```python
from build123d import *

# Parameters (mm, degrees)
SKETCH_1_W          = 27.799055089
SKETCH_1_H          = 170
SKETCH_1_R          = 1.5
EXTRUDE_1_DEPTH     = 5
EXTRUDE_2_DEPTH     = 170
FILLET_1_R          = 20
FILLET_2_R          = 20
SKETCH_3_R          = 1.5
CUT_EXTRUDE_1_DEPTH = 22
SKETCH_5_W          = 53.411136204
SKETCH_5_H          = 30.531921538
CUT_EXTRUDE_2_DEPTH = 138
SKETCH_6_W          = 16.9901426
SKETCH_6_H          = 53.411136204
EXTRUDE_3_DEPTH     = 7.098148729
FILLET_3_R          = 2
SKETCH_7_R          = 1.5
CUT_EXTRUDE_3_DEPTH = 20


with BuildPart() as part:
    # 草图1 → 凸台-拉伸1 (new body)
    with BuildSketch(Plane(origin=(0, 0, 0), x_dir=(1, 0, 0), z_dir=(0, 1, 0))):
        with Locations((91.881203353, 5)):
            Rectangle(SKETCH_1_W, SKETCH_1_H)
        with Locations(Location((82.140918425, 87.25, 0), (0, 0, 270))):
            Circle(SKETCH_1_R, mode=Mode.SUBTRACT)
        with Locations(Location((92.640918425, 87.25, 0), (0, 0, 270))):
            Circle(SKETCH_1_R, mode=Mode.SUBTRACT)
        with Locations(Location((82.140918425, -77.25, 0), (0, 0, 270))):
            Circle(SKETCH_1_R, mode=Mode.SUBTRACT)
        with Locations(Location((92.640918425, -77.25, 0), (0, 0, 270))):
            Circle(SKETCH_1_R, mode=Mode.SUBTRACT)
    extrude(amount=EXTRUDE_1_DEPTH)

    # 草图2 → 凸台-拉伸2 (add)
    with BuildSketch(Plane.XY.offset(80)):
        Polygon((70.154089187, 3.11568229), (59.601778844, 32.107916678), (60.432470808, 37.577633674), (62.77468262, 53), (74.6026601, 53), (68.115201024, 32.107916678), (77.981675808, 5), (77.981675808, 0), (71.288104799, 0), align=None)
    extrude(amount=-EXTRUDE_2_DEPTH)

    # 圆角1
    fillet_1_edges = [part.edges().sort_by_distance(p)[0] for p in [
        (59.601778844, 32.107916678, -5),
    ]]
    fillet(fillet_1_edges, radius=FILLET_1_R)

    # 圆角2
    # the kernel refuses this fillet: 20 mm, written as the material it takes off along each edge
    with BuildSketch(Plane(origin=(71.288104799, 0, 115.01037691), x_dir=(-0.34202014332567304, 0.9396926207859069, 0), z_dir=(0, 0, -1))) as fillet_2_piece_1:
        with BuildLine():
            CenterArc((FILLET_2_R * 0.70020753821, FILLET_2_R), FILLET_2_R, 200, 70)
            Line((-FILLET_2_R * 0.239485082576, FILLET_2_R * 0.657979856674), (0, 0))
            Line((0, 0), (FILLET_2_R * 0.70020753821, 0))
        make_face()
    extrude(amount=240.020753821, mode=Mode.SUBTRACT)

    # 草图3 → 切除-拉伸1 (cut)
    with BuildSketch(Plane(origin=(0, 53, 0), x_dir=(1, 0, 0), z_dir=(0, 1, 0))):
        with Locations(Location((71.288104799, 70.02483454, 0), (0, 0, 270))):
            Circle(SKETCH_3_R)
        with Locations(Location((65.841750728, 62.078973455, 0), (0, 0, 270))):
            Circle(SKETCH_3_R)
        with Locations(Location((65.841750728, 55.078973455, 0), (0, 0, 270))):
            Circle(SKETCH_3_R)
        with Locations(Location((71.288104799, 47.133112371, 0), (0, 0, 270))):
            Circle(SKETCH_3_R)
        with Locations(Location((71.288104799, -37.133112371, 0), (0, 0, 270))):
            Circle(SKETCH_3_R)
        with Locations(Location((65.841750728, -45.078973455, 0), (0, 0, 270))):
            Circle(SKETCH_3_R)
        with Locations(Location((65.841750728, -52.078973455, 0), (0, 0, 270))):
            Circle(SKETCH_3_R)
        with Locations(Location((71.288104799, -60.02483454, 0), (0, 0, 270))):
            Circle(SKETCH_3_R)
    extrude(amount=-CUT_EXTRUDE_1_DEPTH, mode=Mode.SUBTRACT)

    # 草图5 → 切除-拉伸2 (cut)
    with BuildSketch(Plane(origin=(0, 0, 0), x_dir=(0, 0, -1), z_dir=(1, 0, 0))):
        with Locations((5, 27.364109498)):
            Rectangle(SKETCH_5_W, SKETCH_5_H)
    extrude(amount=CUT_EXTRUDE_2_DEPTH, mode=Mode.SUBTRACT)

    # 草图6 → 凸台-拉伸3 (add)
    with BuildSketch(Plane(origin=(0, 5, 0), x_dir=(1, 0, 0), z_dir=(0, 1, 0))):
        with Locations((83.893232252, 5)):
            Rectangle(SKETCH_6_W, SKETCH_6_H)
    extrude(amount=EXTRUDE_3_DEPTH)

    # 圆角3
    fillet_3_edges = [part.edges().sort_by_distance(p)[0] for p in [
        (71.158795105, 12.098148729, -31.705568102),
        (71.158795105, 12.098148729, 21.705568102),
        (66.291177476, 42.630070267, 21.705568102),
        (66.291177476, 42.630070267, -31.705568102),
    ]]
    fillet(fillet_3_edges, radius=FILLET_3_R)

    # 草图7 → 切除-拉伸3 (cut)
    with BuildSketch(Plane(origin=(0, 12.098148729, 0), x_dir=(1, 0, 0), z_dir=(0, 1, 0))):
        with Locations(Location((71.530354556, -14, 0), (0, 0, 270))):
            Circle(SKETCH_7_R)
        with Locations(Location((71.530354556, 24, 0), (0, 0, 270))):
            Circle(SKETCH_7_R)
        with Locations(Location((86.530354556, 24, 0), (0, 0, 270))):
            Circle(SKETCH_7_R)
        with Locations(Location((86.530354556, -14, 0), (0, 0, 270))):
            Circle(SKETCH_7_R)
    extrude(amount=-CUT_EXTRUDE_3_DEPTH, mode=Mode.SUBTRACT)


solid = part.part
```
Can you work these out from the model? Positions are in its coordinate system, mm. A direction names the side the tool comes from. Give positions to 0.01 mm unless a question says otherwise; leave off trailing zeros. Write each loop counter-clockwise with the first axis right and the second up, starting at its lowest first coordinate (ties: lowest second). Pieces come first, ordered by that corner, then holes. Notation, with made-up numbers: (74, 24) -> (133, 24) arc R15 ccw to (133, 37) -> close; hole circle Ø4 at (26, -36.75). An arc over 180 degrees is marked (long way). One line per item, written item: value.
Q1. Imagine slicing it at B-B on z = 77.25. Please give me the cut outline in (x, y).
Results found:
outline: (60.37, 37.15) arc R20 ccw to (61.35, 27.31) -> (66.5, 13.16) arc R20 ccw to (80.64, 0.55) -> (80.64, 5) -> (77.98, 5) -> (68.12, 32.11) -> (74.6, 53) -> (62.77, 53) -> close; (83.64, 0.07) arc R20 ccw to (85.29, 0) -> (91.14, 0) -> (91.14, 5) -> (83.64, 5) -> close; (94.14, 0) -> (105.78, 0) -> (105.78, 5) -> (94.14, 5) -> close
Q2. Imagine slicing it at A-A on y = 46. Please give me the cut outline in (x, z).
Results found:
outline: (61.71, -90) -> (72.43, -90) -> (72.43, -71) arc R1.5 cw (long way) to (72.43, -69.05) -> (72.43, -48.11) arc R1.5 cw (long way) to (72.43, -46.16) -> (72.43, 36.16) arc R1.5 cw (long way) to (72.43, 38.11) -> (72.43, 59.05) arc R1.5 cw (long way) to (72.43, 61) -> (72.43, 80) -> (61.71, 80) -> close; hole circle Ø3 at (65.84, -62.08); hole circle Ø3 at (65.84, -55.08); hole circle Ø3 at (65.84, 45.08); hole circle Ø3 at (65.84, 52.08)
Q3. Which directions (+Z, -Z, +X, -X, +Y, -Y) give clear straight access to the entire face, cutting with the end or side of a thin tool? Please do faces 1 (the face through (60.247, 32.102, 50.445)), 2 (the face through (73.018, 9.082, 13.805)), 3 (the face through (84, 8, 21.706)), 4 (the face through (64.51, 42.15, 45.77)).
Results found:
face 1: +Z, -Z, -X
face 2: -Y
face 3: +Z, +X, +Y
face 4: +Y
Q4. Imagine slicing it at C-C on x = 96. Please give me the cut outline in (y, z).
Results found:
outline: (0, -90) -> (5, -90) -> (5, 80) -> (0, 80) -> close
Q5. Imagine slicing it at D-D on y = 9. Please give me the cut outline in (x, z), and give its area (3 significant figures).
Results found:
outline: (68.59, -90) -> (76.53, -90) -> (76.53, -31.71) -> (92.39, -31.71) -> (92.39, 21.71) -> (76.53, 21.71) -> (76.53, 80) -> (68.59, 80) -> close; hole circle Ø3 at (71.53, -24); hole circle Ø3 at (71.53, 14); hole circle Ø3 at (86.53, -24); hole circle Ø3 at (86.53, 14)
area: 2,170 mm^2
Q6. We'd pull the mould along X, two halves only. Please class faces 5 (the face through (66, 27, -31.706)), 6 (the face through (63.959, 20.136, 51.146)), 7 (the face through (83.628, 2.5, 77.055)), 8 (the face through (72.125, 45.022, -3.81)): +X half, -X half, draft (parallel to the pull), parting line (faces both ways), or undercut.
Results found:
face 5: draft
face 6: -X half
face 7: undercut
face 8: +X half
Q7. Please list where these lines run through material, in increasing order: line 1 (Z direction, x = 68.5, y = 36); line 2 (Z direction, x = 65.5, y = 41); line 3 (Y direction, x = 67.5, z = 2). Write a range as [from, to].
Results found:
line 1: z = [-90, -31.71], [21.71, 80]
line 2: z = [-90, -63.54], [-60.62, -56.54], [-53.62, -31.67], [21.67, 43.62], [46.54, 50.62], [53.54, 80]
line 3: y = [10.87, 12.1], [42.63, 53]
Q8. For P1, Ø1, axis at y = 45, z = 23, coming from the -X side; P2, Ø2.5, axis at x = 92.64, z = 77.25, coming from the -Y side; P3, Ø4, axis at x = 71.29, z = 37.13, coming from the -Y side; P4, Ø5, axis at x = 67.5, z = -11, coming from the -Y side, each with a flat end and sliding along its axis, tell me the tip position at first contact or that it passes through.
Results found:
P1: stops at x = 61.48
P2: passes through
P3: stops at y = 4
P4: stops at y = 7.11
